Can you work these out from the model? Positions are in its coordinate system, mm. A direction names the side the tool comes from. Round coordinates to 2 decimals unless told otherwise and drop trailing zeros. Write each loop counter-clockwise with the first axis right and the second up, starting at its lowest first coordinate (ties: lowest second). Pieces come first, ordered by that corner, then holes. Notation, with made-up numbers: M 74,89 L 116,89 A21 cw 116,96 Z; hole C 62,51.5 d9. An arc over 180 degrees is marked long. Answer in a Markdown table with one row per item. Add a question column.
(1) Suppose I cut it at D-D, the plane z = -9.5. Write out the boundary of the cut face in (x, y).
(2) I'm going to push flat-ended pins straight in: pin 1 (12 mm diameter, centred on y = -0.5, z = -15.5, fed in from +X); pin 2 (3 mm diameter, centred on x = -1, z = -13.5, fed in from +Y); pin 3 (3 mm diameter, centred on y = -6, z = -12.5, fed in from -X). Where does each tip first touch, or does it pass through?
(3) For faces 1 (the face through (-5.723, -1.802, -13.168)), 2 (the face through (0, 0, -29)), 3 (the face through (-2, 0, -31)), which set-ups out of +Z, -Z, +X, -X, +Y, -Y let a thin tool reach every point of the face, with its end or its side?
(4) Suppose I cut it at A-A, the plane y = 0. Write out the boundary of the cut face in (x, z), then the cut area to 3 significant figures.
(5) If we mould it in two halves opening along Y, with no side actions, what happens to faces 4 (the face through (1.382, 6.224, -25.375)), 5 (the face through (0, 1, -30)), 6 (the face through (0, 0, 0))? For each: released by +Y, released by -Y, zero draft, split by the parting line, or undercut.
(6) If I drill on probe 1 along Y at (x, z) = (0, -30.05); probe 2 along Y at (x, z) = (0, -29.4); probe 3 along Z at (x, y) = (-0.75, -0.5), over which ranges is the centre line in solid material (lowest first)?
(7) Suppose I cut it at C-C, the plane z = -28.5. Write out the boundary of the cut face in (x, y), then the cut area to 3 significant figures.
from build123d import *

# Parameters (mm, degrees)
CHAMFER1_SIZE = 1


with BuildPart() as part:
    # Sketch1 → Revolve1 (revolve)
    with BuildSketch(Plane(origin=(0, 0, 0), x_dir=(1, 0, 0), z_dir=(0, 1, 0)), mode=Mode.PRIVATE) as revolve1_sk:
        Polygon((6, 0), (6, 25), (12, 31), (1, 31), (1, 29), (0, 29), (0, 0), align=None)
    revolve(revolve1_sk.sketch.rotate(Axis((0, 0, -48.72611465), (0, 0, 1)), 180), axis=Axis((0, 0, -48.72611465), (0, 0, 1)))

    # Chamfer1
    chamfer1_edges = [part.edges().sort_by_distance(p)[0] for p in [
        (6, 0, 0),
    ]]
    chamfer(chamfer1_edges, length=CHAMFER1_SIZE)


solid = part.part
Calculated:
| question | item | result |
|---|---|---|
| 1 | outline | C 0,0 d12 |
| 2 | pin 1 | x = 6 |
| 2 | pin 2 | y = 6 |
| 2 | pin 3 | x = -3.97 |
| 3 | face 1 | +Z |
| 3 | face 2 | -Z |
| 3 | face 3 | -Z, +X, -X, +Y, -Y |
| 4 | outline | M -12,-31 L -1,-31 L -1,-29 L 1,-29 L 1,-31 L 12,-31 L 6,-25 L 6,-1 L 5,0 L -5,0 L -6,-1 L -6,-25 Z |
| 4 | area | 403 mm² |
| 5 | face 4 | split by the parting line |
| 5 | face 5 | undercut |
| 5 | face 6 | zero draft |
| 6 | probe 1 | -11.05 to -1, 1 to 11.05 |
| 6 | probe 2 | -10.4 to -1, 1 to 10.4 |
| 6 | probe 3 | -29 to 0 |
| 7 | outline | C 0,0 d19 |
| 7 | area | 284 mm² |
